from build123d import *

# Parameters (mm, degrees)
F1_DEPTH = 15.24
F2_D     = 2.286
F2_DEPTH = 15.24
F2_TIP   = 0.6867836875
F3_D     = 5.08
F3_DEPTH = 15.24
F3_TIP   = 1.5261859723
F4_DEPTH = 15.24
F0_W     = 74.4793638587
F0_H     = 6.2680644915
F0_H_2   = 5.8993548155
F5_DEPTH = 15.24


with BuildPart() as f1:
    # F0 (on Right) → F1 (new body)
    with BuildSketch(Plane.YZ):
        Polygon((60.8523078263, 8.4471310302), (60.8523078263, -8.4803225473), (73.919005692, -8.4803225473), (73.919005692, -2.2122580558), (148.3983695507, -2.2122580558), (148.3983695507, -8.4803225473), (162.2249782085, -8.4803225473), (162.2249782085, 8.4803225473), (148.3983695507, 8.4803225473), (148.3983695507, 2.5809677318), (73.919005692, 2.5809677318), (73.919005692, 8.4803225473), (61.3453197977, 8.4803225473), align=None)
    extrude(amount=F1_DEPTH)

    # F2
    with Locations(Plane(origin=(0, 0, 0), x_dir=(0, 1, 0), z_dir=(-1, 0, 0))):
        with Locations((68.0196508765, 0)):
            Hole(F2_D / 2, depth=F2_DEPTH)
            with Locations((0, 0, -(F2_DEPTH + F2_TIP / 2))):  # 118° drill point
                Cone(0, F2_D / 2, F2_TIP, mode=Mode.SUBTRACT)

    # F3
    with Locations(Plane(origin=(0, 0, 0), x_dir=(0, 1, 0), z_dir=(-1, 0, 0))):
        with Locations((156.2374085188, 0)):
            Hole(F3_D / 2, depth=F3_DEPTH)
            with Locations((0, 0, -(F3_DEPTH + F3_TIP / 2))):  # 118° drill point
                Cone(0, F3_D / 2, F3_TIP, mode=Mode.SUBTRACT)

    # F0 (on Right) → F4 (join)
    with BuildSketch(Plane.YZ):
        Polygon((-64.6176040173, 0), (-64.6176040173, -8.4803225473), (-54.0782185303, -8.4803225473), (-54.0782185303, 0.7095531421), align=None)
        Polygon((-54.0782185303, 0.7095531421), (-54.0782185303, -8.4803225473), (-13.8418450952, -8.4803225473), (-13.8418450952, 3.4184250429), align=None)
        Polygon((-13.8418450952, 3.4184250429), (-13.8418450952, -8.4803225473), (-9.9811125547, -8.4803225473), (-9.9811125547, 3.6783448369), align=None)
        Polygon((-9.9811125547, 3.6783448369), (-9.9811125547, -8.4803225473), (20.5496044121, -8.4803225473), (20.5496044121, 5.7337935327), align=None)
        Polygon((24.1768896074, 5.9779967275), (24.1768896074, -8.4803225473), (60.8523078263, -8.4803225473), (60.8523078263, 8.4471310302), align=None)
        Polygon((20.5496044121, 5.7337935327), (20.5496044121, -8.4803225473), (24.1768896074, -8.4803225473), (24.1768896074, 5.9779967275), align=None)
    extrude(amount=F4_DEPTH)

    # F0 (on Right) → F5 (join)
    with BuildSketch(Plane.YZ):
        with Locations((111.1586876214, -5.3462903015)):
            Rectangle(F0_W, F0_H)
        with Locations((111.1586876214, 5.5306451395)):
            Rectangle(F0_W, F0_H_2)
    extrude(amount=F5_DEPTH)


solid = f1.part
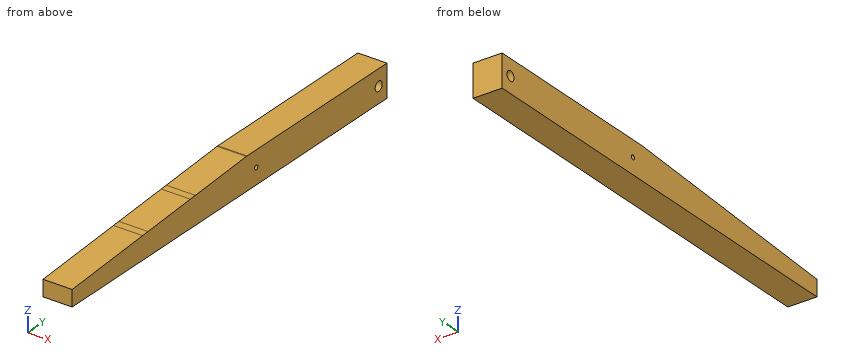
Geometry: final body of the model. Coordinates: model frame, mm. Round coordinates to 2 decimals unless told otherwise and drop trailing zeros. Order: outer loops, then holes, each group sorted by start corner. A loop starts at its lowest first (then second) coordinate and runs counter-clockwise, first axis right, second up. Notation, with made-up numbers: (22.25, -21.5) -> (71.25, -21.5) arc R9 cw to (71.25, -17.5) -> close; hole circle Ø3 at (1.5, -39). An arc over 180 degrees is marked (long way). Put each result on its own line as item: value. Start each with the question number.
Q1. Section B-B on y = 5.5. Return the cut outline in (x, z).
Q2. Section A-A on x = 8.25. Return the cut outline in (y, z).
Q3. Section C-C on y = 29.5. Return the cut outline in (x, z).
Q4. First-contact query: pin 1 (5 mm diameter, centred on y = 3, z = 4.5, fed in from -X); pin 2 (8 mm diameter, centred on x = 4, y = 40, fed in from +Z); pin 3 (8 mm diameter, centred on x = 4, y = -24.5, fed in from +Z); pin 4 (4 mm diameter, centred on y = 156.24, z = 0, fed in from -X). Flat tips, straight axial feed; report the tip coordinate or a pass-through.
Q5. Line query: probe 1 along Y at (x, z) = (6.75, -0.5); probe 2 along Z at (x, y) = (14.25, -47); probe 3 along Z at (x, y) = (9.5, 12.5). Output: solid intervals per line, ascending.
Ans:
1. outline: (0, -8.48) -> (15.24, -8.48) -> (15.24, 4.72) -> (0, 4.72) -> close
2. outline: (-64.62, -8.48) -> (162.22, -8.48) -> (162.22, 8.48) -> (61.35, 8.48) -> (-64.62, 0) -> close; hole circle Ø2.29 at (68.02, 0); hole circle Ø5.08 at (156.24, 0)
3. outline: (0, -8.48) -> (15.24, -8.48) -> (15.24, 6.34) -> (0, 6.34) -> close
4. pin 1: stops at x = 0
4. pin 2: stops at z = 7.31
4. pin 3: stops at z = 2.97
4. pin 4: passes through
5. probe 1: y = -64.62 to 66.99, 69.05 to 153.75, 158.73 to 162.22
5. probe 2: z = -8.48 to 1.19
5. probe 3: z = -8.48 to 5.19
